For this review, use the dimensioned drawing (mm, ordinates from the lowest corner) and the shaded views. A direction names the side the tool comes from. Round coordinates to 2 decimals unless told otherwise and drop trailing zeros. Loops run counter-clockwise (first coordinate to the right, second up) from the corner with the lowest first, then second, coordinate; pieces in that order, holes last. Notation, with made-up numbers: M 31.5,13.25 L 68.5,13.25 A22 cw 68.5,24.25 Z; hole C 42.25,57.25 d9. An arc over 180 degrees is marked long. Answer as a JSON object with one key per item and string values. Group by question number.
Item 1: Tool access review of the marked faces 4, 5 and 6: name each direction out of +Z, -Z, +X, -X, +Y, -Y from which nothing blocks a thin tool from reaching the whole face with its end or side.
Item 2: Consider section A-A (x = 140). Give the boundary of the cut face in (y, z).
Item 3: Consider section B-B (y = 70). Give the boundary of the cut face in (x, z).
Item 4: The part is to be moulded in two halves that separate along Y. For the marked faces 1, 2 and 3, say which applies: +Y half, -Y half, draft (parallel to the pull), parting line (faces both ways), or undercut.
Item 5: Insertion check: P1, Ø7.5, axis at x = 2.5, z = 5, coming from the +Y side; P2, Ø3.5, axis at x = 3.5, z = 10.5, coming from the -Y side; P3, Ø2, axis at y = 82.5, z = 6.5, coming from the -X side. Each pin has a flat end and moves straight along its axis. Give the tip position at first contact, or say it passes through.
Item 6: Consider section D-D (x = 182). Give the boundary of the cut face in (y, z).
Item 7: Consider section C-C (z = 6). Give the boundary of the cut face in (x, y), and give its area (3 significant figures).
Item 8: To check wall thickness, follow line 1 (Y direction, x = 77.5, z = 14); line 2 (Z direction, x = 12, y = 66); line 3 (Z direction, x = 15, y = 42). State the ranges of each line that lie inside material, in increasing order.
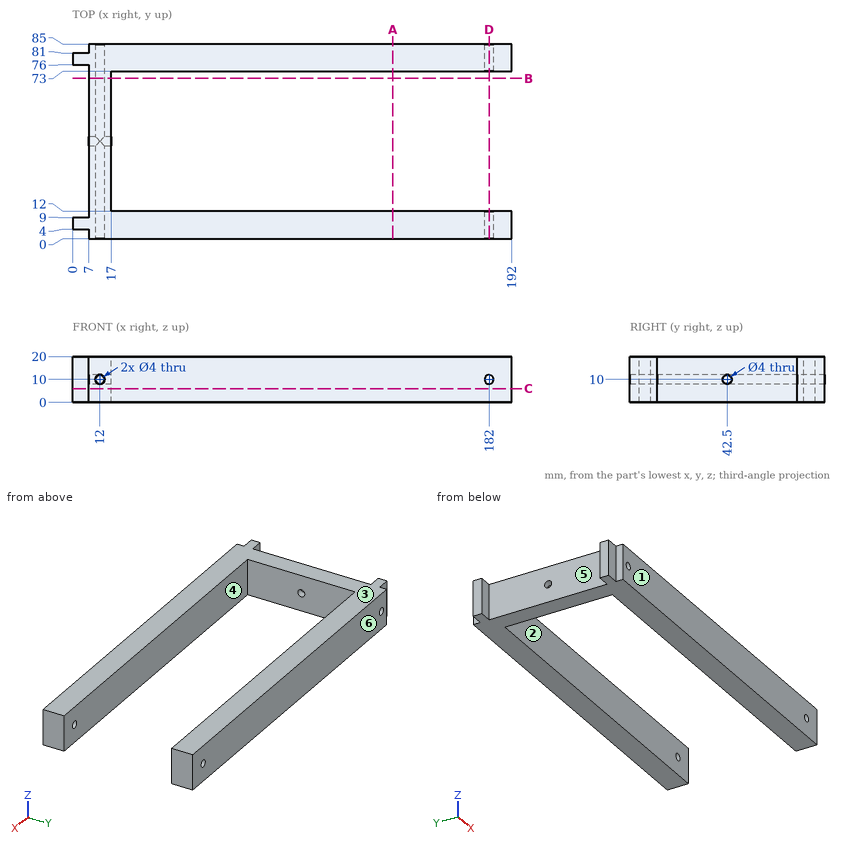
Geometry results:
{
 "1": {"face 4": "+Z, -Z, +X", "face 5": "+Z, -Z, -X", "face 6": "+Z, -Z, +X, -X, +Y"},
 "2": {"outline": "M 0,0 L 12,0 L 12,20 L 0,20 Z; M 73,0 L 85,0 L 85,20 L 73,20 Z"},
 "3": {"outline": "M 7,0 L 17,0 L 17,20 L 7,20 Z; hole C 12,10 d4"},
 "4": {"face 1": "-Y half", "face 2": "undercut", "face 3": "draft"},
 "5": {"P1": "stops at y = 81", "P2": "stops at y = 4", "P3": "stops at x = 7"},
 "6": {"outline": "M 0,0 L 12,0 L 12,8 L 0,8 Z; M 0,12 L 12,12 L 12,20 L 0,20 Z; M 73,0 L 85,0 L 85,8 L 73,8 Z; M 73,12 L 85,12 L 85,20 L 73,20 Z"},
 "7": {"outline": "M 0,4 L 7,4 L 7,0 L 192,0 L 192,12 L 17,12 L 17,73 L 192,73 L 192,85 L 7,85 L 7,81 L 0,81 L 0,76 L 7,76 L 7,9 L 0,9 Z", "area": "5,120 mm^2"},
 "8": {"line 1": "y = 0 to 12, 73 to 85", "line 2": "z = 0 to 8, 12 to 20", "line 3": "z = 0 to 8.06, 11.94 to 20"}
}
